Check sheet for the drawn part. Datum: minimum x, y, z corner. Units: mm. Round coordinates to 2 decimals unless told otherwise and drop trailing zeros. Write each loop counter-clockwise with the first axis right and the second up, starting at its lowest first coordinate (ties: lowest second). Pieces come first, ordered by that corner, then holes. Notation, with made-up numbers: M -39,64 L -12,64 A24 ccw -12,93 Z; hole C 75.5,-15 d3. An arc over 180 degrees is marked long. Put each result on its own line as item: value.
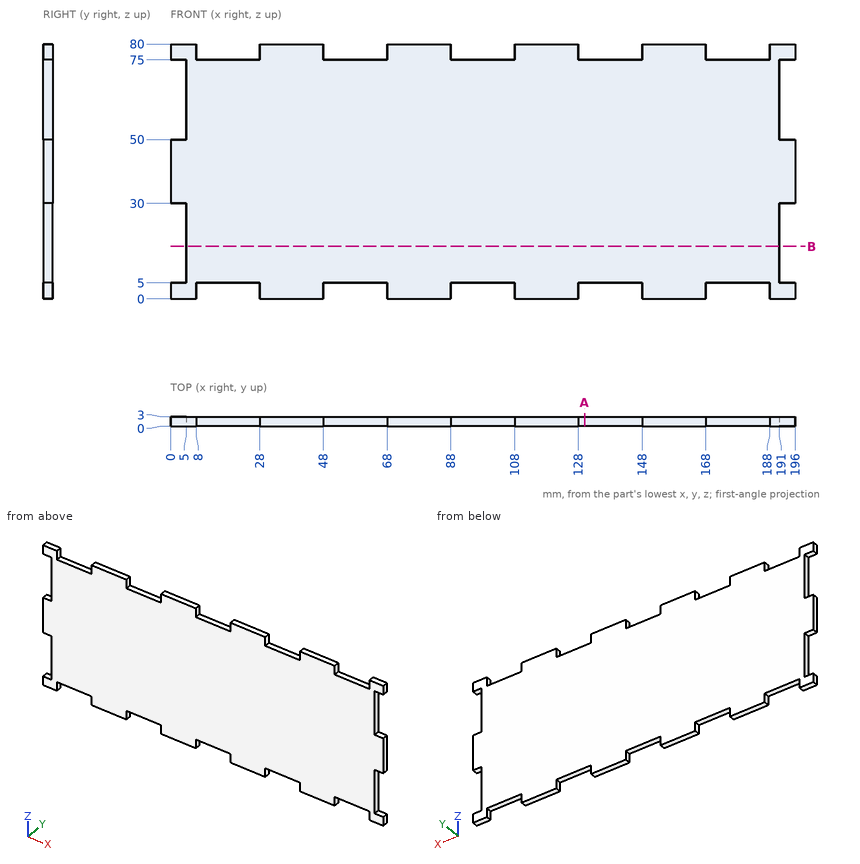
1. Depth check by flat-ended pin: pin 1 Ø0.9 at (x, y) = (54, 2) entering from +Z; pin 2 Ø0.9 at (y, z) = (1.5, 2) entering from -X; pin 3 Ø0.9 at (y, z) = (1.5, 63) entering from +X; pin 4 Ø0.9 at (y, z) = (1, 60) entering from -X. Enter the tip coordinate at first touch or a pass-through.
Computed values:
pin 1: stops at z = 75
pin 2: stops at x = 0
pin 3: stops at x = 191
pin 4: stops at x = 5
2. Cross-section at B-B (z = 16.5). Enter the section's corners in (x, y), then the cut area to 3 significant figures.
Computed values:
outline: M 5,0 L 191,0 L 191,3 L 5,3 Z
area: 558 mm2
3. Cross-section at A-A (x = 130). Enter the section's corners in (y, z), then the cut area to 3 significant figures.
Computed values:
outline: M 0,5 L 3,5 L 3,75 L 0,75 Z
area: 210 mm2
4. Scan lines: probe 1 along X at (y, z) = (1.3, 57); probe 2 along Z at (x, y) = (10.5, 2.45). Record each from-to range of solid material in increasing order.
Computed values:
probe 1: x = 5 to 191
probe 2: z = 5 to 75
